Verification items for this drawing (mm, ordinates from the low corner). A direction names the side the tool comes from. Give positions to 0.01 mm unless a question says otherwise; leave off trailing zeros. Write each loop counter-clockwise with the first axis right and the second up, starting at its lowest first coordinate (ties: lowest second). Pieces come first, ordered by that corner, then holes. Notation, with made-up numbers: (3.25, 12.5) -> (8.25, 12.5) arc R17 ccw to (8.25, 44.5) -> close; hole circle Ø8 at (71, 89). An arc over 180 degrees is marked (long way). One line per item, written item: value.
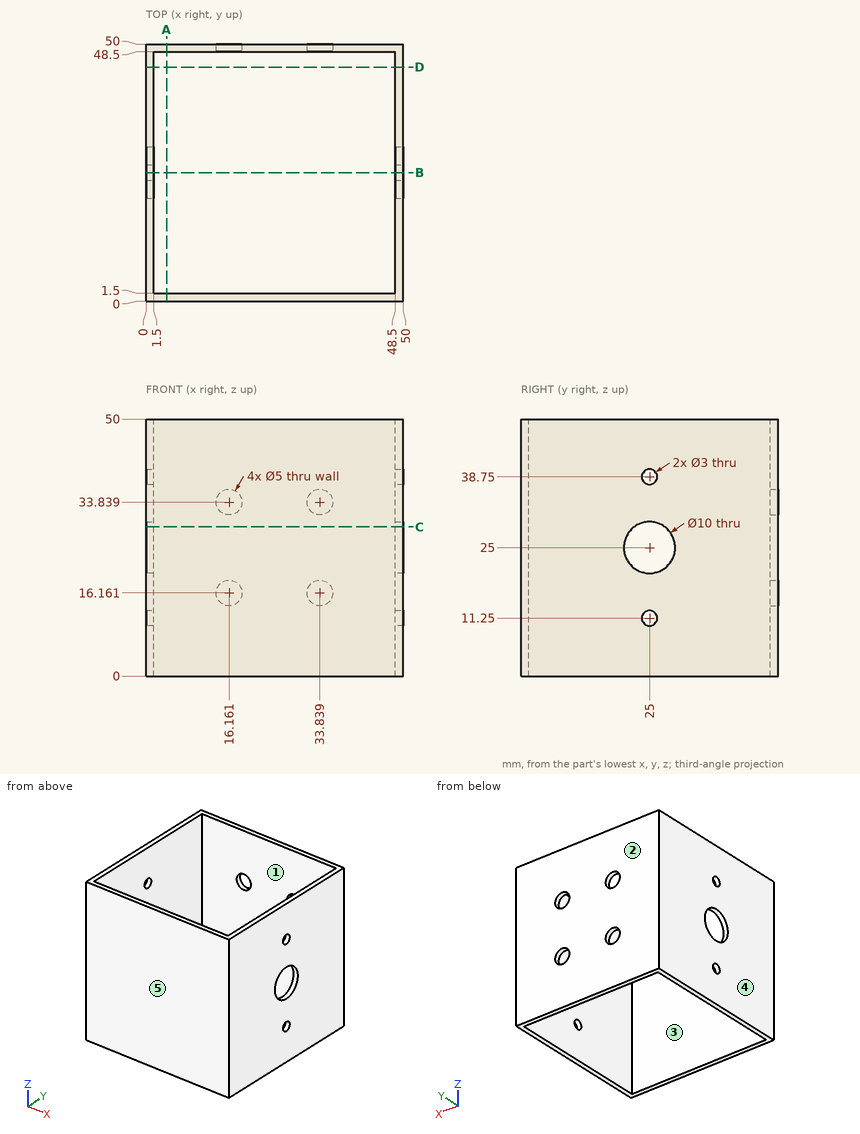
1) Mould release check, pull along Y, two halves, no side actions. Record for the marked faces 3, 4 and 5: released by +Y, released by -Y, zero draft, split by the parting line, or undercut.
Verdict:
face 3: undercut
face 4: zero draft
face 5: released by -Y
2) Sectioned sample at C-C on z = 29. Record the cut outline in (x, y), plus the area to 3 significant figures.
Verdict:
outline: (0, 0) -> (50, 0) -> (50, 22) -> (48.5, 22) -> (48.5, 1.5) -> (1.5, 1.5) -> (1.5, 22) -> (0, 22) -> close; (0, 28) -> (1.5, 28) -> (1.5, 48.5) -> (48.5, 48.5) -> (48.5, 28) -> (50, 28) -> (50, 50) -> (0, 50) -> close
area: 273 mm^2
3) Depth check by flat-ended pin: pin 1 Ø2.5 at (y, z) = (25, 38.75) entering from +X. Enter the tip coordinate at first touch or a pass-through.
Verdict:
pin 1: through
4) Sectioned sample at A-A on x = 4. Record the cut outline in (y, z), plus the area to 3 significant figures.
Verdict:
outline: (0, 0) -> (1.5, 0) -> (1.5, 50) -> (0, 50) -> close; (48.5, 0) -> (50, 0) -> (50, 50) -> (48.5, 50) -> close
area: 150 mm^2
5) Tool access check on the marked faces 1 and 2. Record the directions out of +Z, -Z, +X, -X, +Y, -Y that give a thin tool (end or side, any length) a straight path to the whole face; none if there is none.
Verdict:
face 1: +Z, -Z
face 2: +Z, -Z, +X, -X, +Y
6) Scan lines: probe 1 along Y at (x, z) = (35.5, 41); probe 2 along Y at (x, z) = (49.45, 38.75). Record each from-to range of solid material in increasing order.
Verdict:
probe 1: 0 to 1.5, 48.5 to 50
probe 2: 0 to 23.5, 26.5 to 50
7) Sectioned sample at B-B on y = 25. Give the number of separate pieces and of enclosed holes in the cut face, plus the area to 3 significant figures.
Verdict:
separate pieces: 8
enclosed holes: 0
area: 102 mm^2
